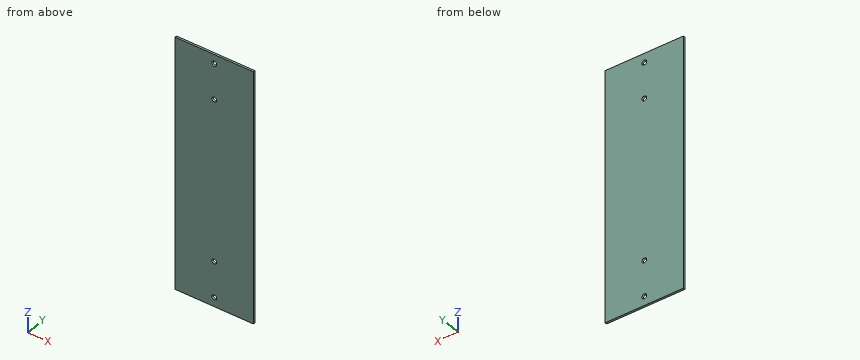
Autodesk Inventor part; units mm, degrees
ref_plane "YZ Plane" through (0, 0, 0) normal (1, 0, 0) x (0, 1, 0)
ref_plane "XZ Plane" through (0, 0, 0) normal (0, 1, 0) x (-1, 0, 0)
ref_plane "XY Plane" through (0, 0, 0) normal (0, 0, 1) x (1, 0, 0)
sketch "スケッチ1" plane through (0, 0, 0) normal (0, 1, 0) x (-1, 0, 0)
  line L0 (0, 0) -> (80, 0)
  line L1 (80, 0) -> (80, -260)
  line L2 (80, -260) -> (0, -260)
  line L3 (0, -260) -> (0, 0)
  dimension "d0" = 80
  dimension "d1" = 260
extrude "押し出し1" add sketch "スケッチ1" along normal blind 2
sketch "スケッチ2" plane through (0, 0, 0) normal (0, -1, 0) x (1, 0, 0)
  circle A0 centre (-40, -9.5) radius 2.5
  line L0 (0, -260) -> (0, 0)
  line L1 (0, 0) -> (-80, 0)
  circle A1 centre (-40, -46.5) radius 2.5
  circle A2 centre (-40, -250.5) radius 2.5
  circle A3 centre (-40, -213.5) radius 2.5
  line L2 (-80, -260) -> (0, -260)
  dimension "d4" = 5
  dimension "d6" = 40
  dimension "d7" = 9.5
  dimension "d8" = 5
  dimension "d10" = 40
  dimension "d11" = 5
  dimension "d12" = 5
  dimension "d13" = 40
  dimension "d14" = 9.5
  dimension "d15" = 40
  dimension "d28" = 37
  dimension "d29" = 37
extrude "押し出し2" cut sketch "スケッチ2" against normal blind 10
Check sheet for the modelled part. Datum: model origin and axes. Units: mm. Round coordinates to 2 decimals unless told otherwise and drop trailing zeros. Loops run counter-clockwise (first coordinate to the right, second up) from the corner with the lowest first, then second, coordinate; pieces in that order, holes last. Notation, with made-up numbers: M 61.25,-29 L 77.25,-29 A9 ccw 77.25,-16 Z; hole C 89.5,67.25 d4. An arc over 180 degrees is marked long. One line per item, written item: value.
(1) Sectioned sample at A-A, the plane z = -9.5. Record the cut outline in (x, y), then the cut area to 3 significant figures.
Computed values:
outline: M -80,0 L -42.5,0 L -42.5,2 L -80,2 Z; M -37.5,0 L 0,0 L 0,2 L -37.5,2 Z
area: 150 mm^2
(2) Depth check by flat-ended pin: pin 1 Ø4 at (x, z) = (-40, -46.5) entering from +Y. Enter the tip coordinate at first touch or a pass-through.
Computed values:
pin 1: passes through
(3) Thickness scan on line 1 (Z direction, x = -40, y = 1); line 2 (Z direction, x = -41.5, y = 0.85). Record the ranges inside material, lowest first.
Computed values:
line 1: z = -260 to -253, -248 to -216, -211 to -49, -44 to -12, -7 to 0
line 2: z = -260 to -252.5, -248.5 to -215.5, -211.5 to -48.5, -44.5 to -11.5, -7.5 to 0
